from build123d import *

# Parameters (mm, degrees)
SKETCH2_R            = 50
BOSS_EXTRUDE1_DEPTH  = 4
BOSS_EXTRUDE2_DEPTH  = 14
CUT_EXTRUDE5_REACH   = 134.235
SKETCH30_R           = 20
BOSS_EXTRUDE12_DEPTH = 5
SKETCH5_R            = 2.5
CUT_EXTRUDE18_DEPTH  = 5
SKETCH4_R            = 1.5
CUT_EXTRUDE19_DEPTH  = 5
SKETCH9_R            = 2
CUT_EXTRUDE6_DEPTH   = 7.5
FILLET7_R            = 5
CUT_EXTRUDE20_DEPTH  = 1.5
SKETCH32_R           = 9
CUT_EXTRUDE21_DEPTH  = 10


with BuildPart() as part:
    # Sketch2 → Boss-Extrude1 (new body)
    with BuildSketch(Plane(origin=(0, 0, 0), x_dir=(1, 0, 0), z_dir=(0, 1, 0))):
        with Locations(Location((0, 0, 0), (0, 0, 270))):
            Circle(SKETCH2_R)
    extrude(amount=BOSS_EXTRUDE1_DEPTH)

    # Sketch7 → Boss-Extrude2 (add)
    with BuildSketch(Plane(origin=(7, 0, 0), x_dir=(0, 0, -1), z_dir=(1, 0, 0))):
        with BuildLine():
            Line((25, 4), (25, 6.428793809))
            ThreePointArc((25, 6.428793809), (26.650688088, 13.958734048), (31.3, 20.107609548))
            Line((31.3, 20.107609548), (66.25, 50.001644808))
            ThreePointArc((66.25, 50.001644808), (68.998355192, 85.25), (33.75, 87.998355192))
            Line((33.75, 87.998355192), (-16.25, 45.23149502))
            ThreePointArc((-16.25, 45.23149502), (-22.707377656, 36.691390159), (-25, 26.233139828))
            Line((-25, 26.233139828), (-25, 4))
            Line((-25, 4), (25, 4))
        make_face()
    extrude(amount=-BOSS_EXTRUDE2_DEPTH)

    # Sketch8 → Cut-Extrude5 (cut, up to next)
    with BuildSketch(Plane(origin=(5, 0, 0), x_dir=(0, 0, -1), z_dir=(1, 0, 0)), mode=Mode.PRIVATE) as cut_extrude5_sk1:
        Polygon((20.224986928, 57.349309181), (51.382289443, 83.999309181), (65.032289443, 68.040690819), (33.874986928, 41.390690819), align=None)
    cut_extrude5_tool1 = extrude(cut_extrude5_sk1.sketch, amount=-CUT_EXTRUDE5_REACH, mode=Mode.PRIVATE) & part.part
    add(cut_extrude5_tool1.solids().sort_by_distance((5, 62.695, -42.628638))[0], mode=Mode.SUBTRACT)

    # Sketch30 → Boss-Extrude12 (add)
    with BuildSketch(Plane.XZ):
        with Locations(Location((0, 0, 0), (0, 0, 270))):
            Circle(SKETCH30_R)
    extrude(amount=BOSS_EXTRUDE12_DEPTH)

    # Sketch5 → Cut-Extrude18 (cut)
    with BuildSketch(Plane.XZ):
        with Locations(Location((0, 0, 0), (0, 0, 270))):
            Circle(SKETCH5_R)
    extrude(amount=CUT_EXTRUDE18_DEPTH, mode=Mode.SUBTRACT)

    # Sketch4 → Cut-Extrude19 (cut)
    with BuildSketch(Plane.XZ):
        with Locations(Location((0, 6, 0), (0, 0, 270))):
            Circle(SKETCH4_R)
        with Locations(Location((0, -6, 0), (0, 0, 270))):
            Circle(SKETCH4_R)
    extrude(amount=CUT_EXTRUDE19_DEPTH, mode=Mode.SUBTRACT)

    # Sketch9 → Cut-Extrude6 (cut)
    with BuildSketch(Plane.ZY.offset(7)):
        with Locations((-65.028980219, 75.275328962)):
            Circle(SKETCH9_R)
        with Locations((-20.228296152, 50.114671038)):
            Circle(SKETCH9_R)
        with Locations((-26.728296152, 42.515328962)):
            Circle(SKETCH9_R)
        with Locations((-58.528980219, 82.874671038)):
            Circle(SKETCH9_R)
    extrude(amount=-CUT_EXTRUDE6_DEPTH, mode=Mode.SUBTRACT)

    # Fillet7
    fillet7_edges = [part.edges().sort_by_distance(p)[0] for p in [
        (-7, 35.054627178, -48.775),
        (7, 85.25, -68.998355192),
        (7, 66.614925106, -8.75),
        (-7, 85.25, -68.998355192),
        (-7, 13.958734048, -26.650688088),
        (-7, 5.214396905, -25),
        (-7, 15.116569914, 25),
        (-7, 66.614925106, -8.75),
        (-7, 36.691390159, 22.707377656),
        (7, 36.691390159, 22.707377656),
        (7, 35.054627178, -48.775),
        (7, 15.116569914, 25),
        (7, 5.214396905, -25),
        (7, 13.958734048, -26.650688088),
    ]]
    fillet(fillet7_edges, radius=FILLET7_R)

    # Sketch31 → Cut-Extrude20 (cut)
    with BuildSketch(Plane.ZY.offset(7)):
        Polygon((-14.525480371, 52.474309181), (-28.175480371, 36.515690819), (-70.731796001, 72.915690819), (-57.081796001, 88.874309181), align=None)
    extrude(amount=-CUT_EXTRUDE20_DEPTH, mode=Mode.SUBTRACT)

    # Sketch32 → Cut-Extrude21 (cut)
    with BuildSketch(Plane(origin=(7, 0, 0), x_dir=(0, 0, -1), z_dir=(1, 0, 0))):
        with Locations((50.227980262, 69.195)):
            Circle(SKETCH32_R)
    extrude(amount=-CUT_EXTRUDE21_DEPTH, mode=Mode.SUBTRACT)


solid = part.part
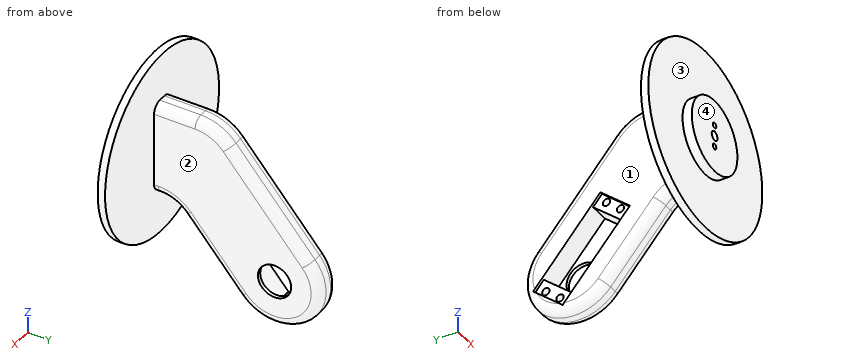
Work out the finished part from the listing and answer in its coordinate system (mm). Face numbers are marked on the shaded views. A direction names the side the tool comes from. Give positions to 0.01 mm unless a question says otherwise; leave off trailing zeros. Order: outer loops, then holes, each group sorted by start corner. A loop starts at its lowest first (then second) coordinate and runs counter-clockwise, first axis right, second up. Notation, with made-up numbers: (73.5, -34.75) -> (82.5, -34.75) arc R6 ccw to (82.5, -29.75) -> close; hole circle Ø11 at (-38.5, 2). An arc over 180 degrees is marked (long way). Answer as a JSON object with one key per item and string values. Group by question number.
1. A tool of negligible diameter and unlimited length cuts with its end or side. For the marked faces 1, 2, 3 and 4, from which of +Z, -Z, +X, -X, +Y, -Y can it reach the whole face along a straight path? Write none if from no direction.
2. Section A-A on x = 32 is taken. Determine the outline of the cut face in (y, z).
3. Section B-B on x = -22 is taken. Determine the outline of the cut face in (y, z).
4. Flat-ended cylindrical pins translate along their axes: pin 1 Ø6 at (x, z) = (24, -50) entering from +Y; pin 2 Ø5 at (x, z) = (23, 2.5) entering from -Y; pin 3 Ø2 at (y, z) = (82.5, -59) entering from -X; pin 4 Ø10 at (x, y) = (-5.5, 14) entering from +Z. Find the tip coordinate at first contact, or state that the pin passes through.
5. Consider line 1 along X through (y, z) = (79, -37); line 2 along Y through (x, z) = (31.5, 18.5); line 3 along Z through (x, y) = (3.5, 69.5). Determine where each line is inside the solid, lowest interval first. Write a range as [from, to].
Result sheet:
{
 "1": {"face 1": "+Z, -Z, -X, +Y", "face 2": "+Z, -Z, +X, +Y", "face 3": "-Y", "face 4": "+Z, -Z, +X, -X, -Y"},
 "2": {"outline": "(0, -38.42) -> (4, -38.42) -> (4, 38.42) -> (0, 38.42) -> close"},
 "3": {"outline": "(0, -44.9) -> (4, -44.9) -> (4, 44.9) -> (0, 44.9) -> close"},
 "4": {"pin 1": "passes through", "pin 2": "stops at y = 0", "pin 3": "stops at x = 0.5", "pin 4": "stops at z = 25"},
 "5": {"line 1": "x = [-7, 7]", "line 2": "y = [0, 4]", "line 3": "z = [-74.76, -63.78], [-34.43, -12.48]"}
}
